from build123d import *

# Parameters (mm, degrees)
F0_R      = 9
F1_DEPTH  = 5
F2_R      = 5.85
F2_R_2    = 2.25
F3_DEPTH  = 12
F4_R      = 1.375
F5_DEPTH  = 25
F3_FACE_R = 2.25
F6_DEPTH  = 5
F7_R      = 1.4
F8_DEPTH  = 25
F9_R      = 1


with BuildPart() as f1:
    # F0 (on Top) → F1 (new body)
    with BuildSketch(Plane.XY):
        Circle(F0_R)
    extrude(amount=F1_DEPTH)

    # F2 (on face) → F3 (join)
    with BuildSketch(Plane.XY.offset(5)):
        Circle(F2_R)
        Circle(F2_R_2, mode=Mode.SUBTRACT)
    extrude(amount=F3_DEPTH)

    # F4 (on Front) → F5 (cut)
    with BuildSketch(Plane.XZ):
        with Locations((0, 11)):
            Circle(F4_R)
    extrude(amount=-F5_DEPTH, mode=Mode.SUBTRACT)

    # F3_face (on face) → F6 (cut, through all)
    with BuildSketch(Plane.XY.offset(5)):
        Circle(F3_FACE_R)
    extrude(amount=-F6_DEPTH, mode=Mode.SUBTRACT)

    # F7 (on face) → F8 (cut)
    with BuildSketch(Plane(origin=(0, 0, 0), x_dir=(1, 0, 0), z_dir=(0, 0, -1))):
        with Locations((-4.871393, -2.8125)):
            Circle(F7_R)
        with Locations((0, 5.625)):
            Circle(F7_R)
        with Locations((4.871393, -2.8125)):
            Circle(F7_R)
    extrude(amount=-F8_DEPTH, mode=Mode.SUBTRACT)

    # F9
    f9_edges = [f1.edges().sort_by_distance(p)[0] for p in [
        (-9, 0, 5),
    ]]
    fillet(f9_edges, radius=F9_R)


solid = f1.part
Geometry: final body of the model. Coordinates: model frame, mm. A direction names the side the tool comes from. Coordinates: 2 decimals unless noted, no trailing zeros. Order: outer loops, then holes, each group sorted by start corner. A loop starts at its lowest first (then second) coordinate and runs counter-clockwise, first axis right, second up.
1) Section C-C (z = 3.75). Give the number of separate pieces and of enclosed holes in the cut face, then the cut area to 3 significant figures.
Result sheet:
separate pieces: 1
enclosed holes: 4
area: 220 mm2
2) First-contact query: P1, Ø10, axis at x = -1, z = 15, coming from the -Y side; P2, Ø2, axis at x = 4.87, y = 2.81, coming from the +Z side; P3, Ø1.5, axis at y = 1, z = 13.5, coming from the -X side; P4, Ø5, axis at x = -3.5, z = 10.5, coming from the +Y side. Flat tips, straight axial feed; report the tip coordinate or a pass-through.
Result sheet:
P1: stops at y = -5.68
P2: passes through
P3: stops at x = -5.84
P4: stops at y = 5.76
3) Ray query, probe 1 along Y at (x, z) = (0, 7.5) (3 decimals); probe 2 along Z at (x, y) = (-1, 6.25); probe 3 along X at (y, z) = (1.75, 4.5). Return the intervals inside material, ascending.
Result sheet:
probe 1: y = -4.225 to -2.25, 2.25 to 5.85
probe 2: z = 0 to 5
probe 3: x = -8.69 to -5.78, -3.96 to -1.41, 1.41 to 3.96, 5.78 to 8.69
4) Draft query along Y for faces 4 (the cylindrical face through (-0.977, 5.768, 9.583)), 5 (the cylindrical face through (-4.12, 1.63, 6.49)), 6 (the cylindrical face through (-1.172, 8.923, 1.972)), 7 (the flat face through (-0.1, -2.4, 17)). Return one class per face: released by +Y, released by -Y, zero draft, split by the parting line, or undercut.
Result sheet:
face 4: released by +Y
face 5: undercut
face 6: split by the parting line
face 7: zero draft
5) Set-up query: faces 1 (the flat face through (4, 5, 5)), 2 (the cylindrical face through (-5.099, -2.868, 10.916)), 3 (the cylindrical face through (5.033, -2.982, 10.916)). Return all of +Z, -Z, +X, -X, +Y, -Y with unobstructed straight access to the full face (end or side cutting, diameter ignored); none if empty.
Result sheet:
face 1: +Z
face 2: +Z, -X
face 3: +Z, +X
6) Section A-A (x = 0). Return loops of the section in (y, z) (3 decimals).
Result sheet:
outline: (-9, 0) - (-7.025, 0) - (-7.025, 5) - (-8, 5) arc R1 ccw to (-9, 4) - close; (-4.225, 0) - (-2.25, 0) - (-2.25, 17) - (-4.225, 17) - close; (2.25, 0) - (9, 0) - (9, 4) arc R1 ccw to (8, 5) - (5.85, 5) - (5.85, 9.625) - (2.25, 9.625) - close; (2.25, 12.375) - (5.85, 12.375) - (5.85, 17) - (2.25, 17) - close
